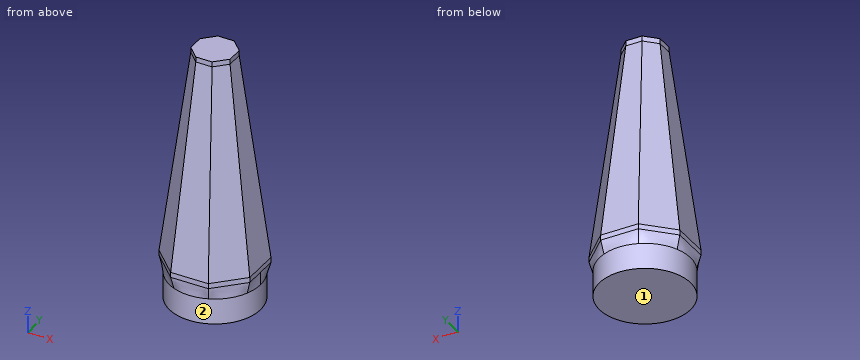
```python
from build123d import *

# Parameters (mm, degrees)
F0_R      = 17.625
F1_DEPTH  = 10
F3_START  = 5
F3_DEPTH  = 2
F6_DEPTH  = 2
F1_FACE_R = 17.625


# Not quite as in the source:
# - a feature names something its author has since deleted; it is built from what else it names


with BuildPart() as f1:
    # F0 (on Top) → F1 (new body)
    with BuildSketch(Plane.XY):
        Circle(F0_R)
    extrude(amount=F1_DEPTH)



with BuildPart() as f3:
    # F2 (on face) → F3 (new body)
    with BuildSketch(Plane.XY.offset(10).offset(F3_START)):
        Polygon((7.3588174532, -17.6007367997), (17.6490700676, -7.2421306223), (17.6007367997, 7.3588174532), (7.2421306223, 17.6490700676), (-7.3588174532, 17.6007367997), (-17.6490700676, 7.2421306223), (-17.6007367997, -7.3588174532), (-7.2421306223, -17.6490700676), align=None)
    extrude(amount=F3_DEPTH)



with BuildPart() as f6:
    # F5 (on offset) → F6 (new body)
    with BuildSketch(Plane.XY.offset(97)):
        Polygon((-7.6354132917, 3.1331203401), (-7.6145031545, -3.1836018769), (-3.1331203401, -7.6354132917), (3.1836018769, -7.6145031545), (7.6354132917, -3.1331203401), (7.6145031545, 3.1836018769), (3.1331203401, 7.6354132917), (-3.1836018769, 7.6145031545), align=None)
    extrude(amount=F6_DEPTH)


with BuildPart() as f3_1:
    add(f3.part)

    add(f6.part)  # F7 merges F6
    # F3_face (on face) → F7 section 0
    with BuildSketch(Plane.XY.offset(17)):
        Polygon((-17.6007367997, -7.3588174532), (-7.2421306223, -17.6490700676), (7.3588174532, -17.6007367997), (17.6490700676, -7.2421306223), (17.6007367997, 7.3588174532), (7.2421306223, 17.6490700676), (-7.3588174532, 17.6007367997), (-17.6490700676, 7.2421306223), align=None)
    # F6_face (on face) → F7 section 1
    with BuildSketch(Plane(origin=(0, 0, 97), x_dir=(1, 0, 0), z_dir=(0, 0, -1))):
        Polygon((-3.1836018769, -7.6145031545), (3.1331203401, -7.6354132917), (7.6145031545, -3.1836018769), (7.6354132917, 3.1331203401), (3.1836018769, 7.6145031545), (-3.1331203401, 7.6354132917), (-7.6145031545, 3.1836018769), (-7.6354132917, -3.1331203401), align=None)
    loft()


with BuildPart() as f1_1:
    add(f1.part)

    add(f3_1.part)  # F8 merges F3
    # F3_face1 (on face) → F8 section 0
    with BuildSketch(Plane(origin=(0, 0, 15), x_dir=(1, 0, 0), z_dir=(0, 0, -1))):
        Polygon((-7.2421306223, 17.6490700676), (-17.6007367997, 7.3588174532), (-17.6490700676, -7.2421306223), (-7.3588174532, -17.6007367997), (7.2421306223, -17.6490700676), (17.6007367997, -7.3588174532), (17.6490700676, 7.2421306223), (7.3588174532, 17.6007367997), align=None)
    # F1_face (on face) → F8 section 1
    with BuildSketch(Plane.XY.offset(10)):
        Circle(F1_FACE_R)
    loft()


solid = f1_1.part
```
The listing builds one solid part. Answer for the finished solid, in the listing's coordinates (mm). Face numbers are marked on the shaded views. A direction names the side the tool comes from. Give positions to 0.01 mm unless a question says otherwise; leave off trailing zeros. Write item = value, one per line. Start each with the question number.
1) Straight lines are drawn through the part: line 1 along Y through (x, z) = (-4, 17); line 2 along X through (y, z) = (7, 63). For each, find the intervals that lie inside material, in ascending order.
2) Which of the six approach directions +Z, -Z, +X, -X, +Y, -Y give full straight-line access (tool end or side, diameter ignored) to the marked faces 1 and 2?
3) Each of these flat-tipped pins is pushed along its axis until it touches: pin 1 (8 mm diameter, centred on y = 11.5, z = 28, fed in from +X); pin 2 (8 mm diameter, centred on y = -7, z = 65.5, fed in from +X); pin 3 (4 mm diameter, centred on x = 13.5, z = 38, fed in from -Y). Where does it stop, or does it pass through?
Solutions:
q1.line_1 = -17.64 to 17.61
q1.line_2 = -9.78 to 9.8
q2.face_1 = -Z, +X, -X, +Y, -Y
q2.face_2 = -Z
q3.pin_1 = 15.57
q3.pin_2 = 12.01
q3.pin_3 = -9.74
